Source: three-view drawing plus pictorial views. Frame: mm from the lowest corner of the part. A direction names the side the tool comes from. Round coordinates to 2 decimals unless told otherwise and drop trailing zeros. Write each loop counter-clockwise with the first axis right and the second up, starting at its lowest first coordinate (ties: lowest second). Pieces come first, ordered by that corner, then holes.
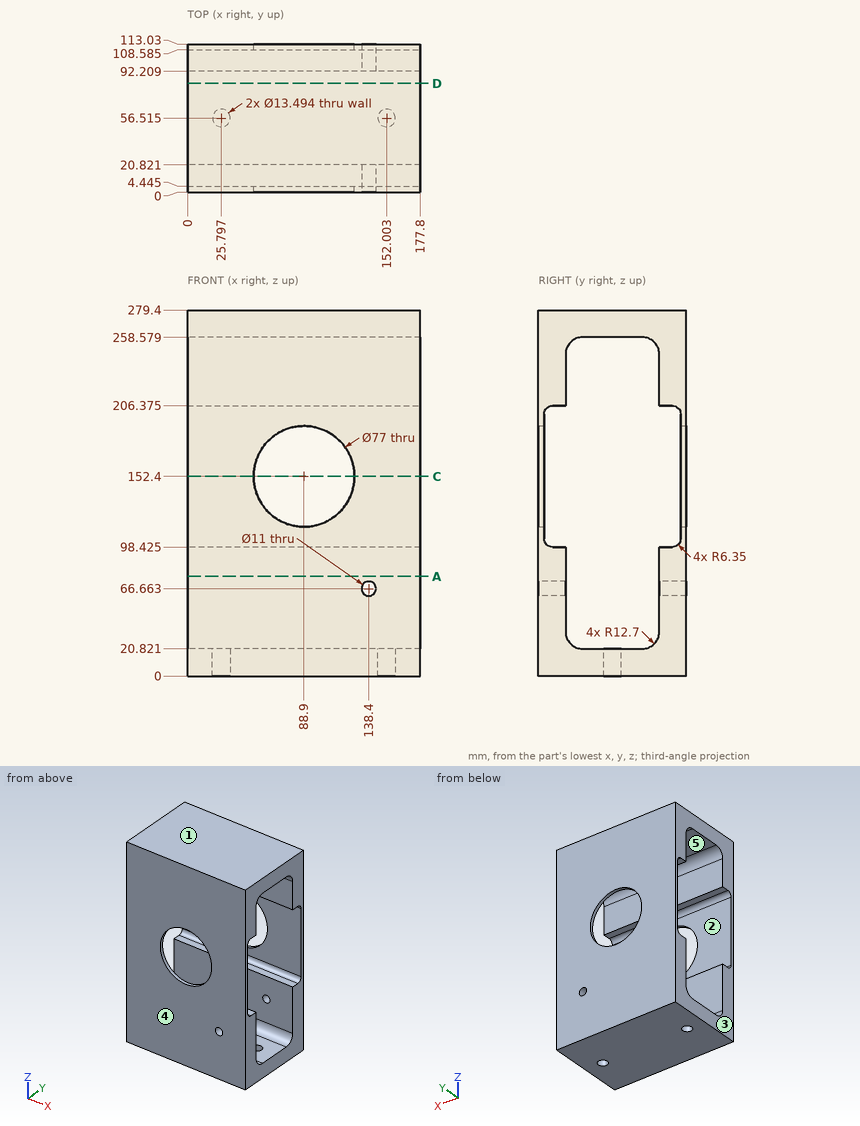
1) Section C-C on z = 152.4. Output: boundary loops of the cut face in (x, y) (1 decimal).
2) Line query: probe 1 along Y at (x, z) = (159, 244); probe 2 along Z at (x, y) = (138.4, 103); probe 3 along Y at (x, z) = (162, 148.5) (1 decimal). Output: solid intervals per line, ascending.
3) Draft query along Z for the marked faces 1, 2 and 3. Return one class per face: pulls with the +Z half, pulls with the -Z half, needs draft (parallel to the pull), parting line crosses it, or undercut.
4) Section D-D on y = 83. Output: boundary loops of the cut face in (x, z), plus the area to 3 significant figures.
5) Section A-A on z = 76. Output: boundary loops of the cut face in (x, y).
6) First-contact query: P1, Ø8, axis at x = 25.8, y = 56.52, coming from the -Z side; P2, Ø17.5, axis at x = 152, y = 56.52, coming from the -Z side; P3, Ø10, axis at x = 138.4, z = 66.66, coming from the +Y side. Flat tips, straight axial feed; report the tip coordinate or a pass-through.
7) Reachability of the marked faces 4 and 5 from +Z, -Z, +X, -X, +Y, -Y: full face, straight path, thin tool, end or side. Return the list, or none.
Filled in:
1. outline: (0, 0) - (50.4, 0) - (50.4, 4.4) - (0, 4.4) - close; (0, 108.6) - (50.4, 108.6) - (50.4, 113) - (0, 113) - close; (127.4, 0) - (177.8, 0) - (177.8, 4.4) - (127.4, 4.4) - close; (127.4, 108.6) - (177.8, 108.6) - (177.8, 113) - (127.4, 113) - close
2. probe 1: y = 0 to 20.82, 92.21 to 113.03
2. probe 2: z = 0 to 61.16, 72.16 to 98.47, 206.33 to 279.4
2. probe 3: y = 0 to 4.4, 108.6 to 113
3. face 1: pulls with the +Z half
3. face 2: undercut
3. face 3: needs draft
4. outline: (0, 0) - (177.8, 0) - (177.8, 21.31) - (0, 21.31) - close; (0, 258.09) - (177.8, 258.09) - (177.8, 279.4) - (0, 279.4) - close
4. area: 7,580 mm2
5. outline: (0, 0) - (177.8, 0) - (177.8, 20.82) - (0, 20.82) - close; (0, 92.21) - (177.8, 92.21) - (177.8, 113.03) - (0, 113.03) - close
6. P1: stops at z = 258.58
6. P2: stops at z = 0
6. P3: passes through
7. face 4: +Z, -Z, +X, -X, -Y
7. face 5: +X, -X
